The model under review builds one solid part; all positions refer to its coordinate system, in mm. Coordinates: 2 decimals unless noted, no trailing zeros. Write each loop counter-clockwise with the first axis right and the second up, starting at its lowest first coordinate (ties: lowest second). Pieces come first, ordered by that corner, then holes.
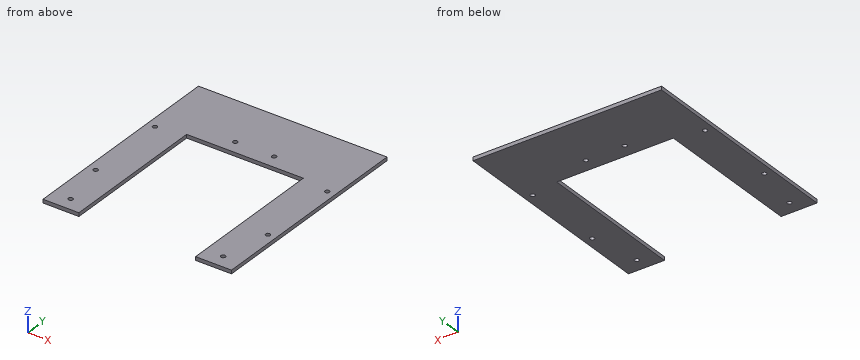
```python
from build123d import *

# Parameters (mm, degrees)
CROQUIS1_R              = 2.5
SALIENTE_EXTRUIR1_DEPTH = 4


with BuildPart() as part:
    # Croquis1 → Saliente-Extruir1 (new body)
    with BuildSketch(Plane.XY):
        Polygon((70, 0), (70, 167), (-60, 167), (-60, 0), (-100, 0), (-100, 241), (110, 241), (110, 0), align=None)
        with Locations((-80, 15)):
            Circle(CROQUIS1_R, mode=Mode.SUBTRACT)
        with Locations((-91, 69.01)):
            Circle(CROQUIS1_R, mode=Mode.SUBTRACT)
        with Locations((-91, 161.01)):
            Circle(CROQUIS1_R, mode=Mode.SUBTRACT)
        with Locations((-16.666666667, 182)):
            Circle(CROQUIS1_R, mode=Mode.SUBTRACT)
        with Locations((26.666666667, 182)):
            Circle(CROQUIS1_R, mode=Mode.SUBTRACT)
        with Locations((101, 161.01)):
            Circle(CROQUIS1_R, mode=Mode.SUBTRACT)
        with Locations((101, 69.01)):
            Circle(CROQUIS1_R, mode=Mode.SUBTRACT)
        with Locations((90, 15)):
            Circle(CROQUIS1_R, mode=Mode.SUBTRACT)
    extrude(amount=SALIENTE_EXTRUIR1_DEPTH)


solid = part.part
```
Item 1: Take a section at A-A, the plane y = 43. Write out the cut boundary in (x, z), plus the area to 3 significant figures.
Solved:
outline: (-100, 0) - (-60, 0) - (-60, 4) - (-100, 4) - close; (70, 0) - (110, 0) - (110, 4) - (70, 4) - close
area: 320 mm2
Item 2: Take a section at C-C, the plane x = -1.5. Write out the cut boundary in (y, z).
Solved:
outline: (167, 0) - (241, 0) - (241, 4) - (167, 4) - close
Item 3: Take a section at B-B, the plane z = 0.6. Count the separate pieces of the cut face and the enclosed holes in it, plus the area to 3 significant figures.
Solved:
separate pieces: 1
enclosed holes: 8
area: 28,700 mm2
Item 4: To check wall thickness, follow line 1 along Y through (x, z) = (-91, 0.35); line 2 along X through (y, z) = (161.01, 3.2); line 3 along X through (y, z) = (130, 1.3). State the ranges of each line that lie inside material, in increasing order.
Solved:
line 1: y = 0 to 66.51, 71.51 to 158.51, 163.51 to 241
line 2: x = -100 to -93.5, -88.5 to -60, 70 to 98.5, 103.5 to 110
line 3: x = -100 to -60, 70 to 110
